```python
from build123d import *

# Parameters (mm, degrees)
SKETCH004_R  = 1.55
PAD005_DEPTH = 0.75
FILLET006_R  = 0.4
FILLET007_R  = 1


with BuildPart() as part:
    # Sketch004 → Pad005 (new body, symmetric)
    with BuildSketch(Plane.XZ):
        with BuildLine():
            Line((-20, 10), (-20, -7))
            Line((-20, -8.5), (-20, -7))
            Line((-20, -8.5), (-20, -10))
            Line((-20, -10), (20, -10))
            Line((20, -10), (20, 4))
            Line((18.133975, 4.5), (20, 4))
            Line((18.133975, 4.5), (-14.2, 4.5))
            ThreePointArc((-15, 4.5), (-14.6, 4.1), (-14.2, 4.5))
            Line((-15, 4.5), (-15, 5.2))
            ThreePointArc((-15, 6), (-15.4, 5.6), (-15, 5.2))
            Line((-15, 6), (18.133975, 6))
            Line((18.133975, 6), (20, 6.5))
            Line((20, 6.5), (20, 10))
            Line((20, 10), (-20, 10))
        make_face()
        Circle(SKETCH004_R, mode=Mode.SUBTRACT)
    extrude(amount=PAD005_DEPTH, both=True)

    # Fillet006
    fillet006_edges = [part.edges().sort_by_distance(p)[0] for p in [
        (-15, 0, 5.2),
        (-14.2, 0, 4.5),
    ]]
    fillet(fillet006_edges, radius=FILLET006_R)

    # Fillet007
    fillet007_edges = [part.edges().sort_by_distance(p)[0] for p in [
        (18.133975, 0, 4.5),
        (18.133975, 0, 6),
        (20, 0, 6.5),
        (20, 0, 10),
        (20, 0, 4),
        (20, 0, -10),
        (-20, 0, -10),
        (-20, 0, 10),
    ]]
    fillet(fillet007_edges, radius=FILLET007_R)


solid = part.part
```
Read the model definition and answer for the solid it produces. Units are mm, in the model's axes. A direction names the side the tool comes from. Coordinates: 2 decimals unless noted, no trailing zeros. Write each loop counter-clockwise with the first axis right and the second up, starting at its lowest first coordinate (ties: lowest second). Pieces come first, ordered by that corner, then holes. Notation, with made-up numbers: (-8.5, 2) -> (40.5, 2) arc R14 cw to (40.5, 15) -> close; hole circle Ø6 at (33.5, -34.75). An arc over 180 degrees is marked (long way). Write item = value, one per line.
(1) Section D-D on x = 16.5 is taken. Write down the section's boundary in (y, z), plus the area to 4 significant figures.
From the geometry:
outline = (-0.75, -10) -> (0.75, -10) -> (0.75, 4.5) -> (-0.75, 4.5) -> close; (-0.75, 6) -> (0.75, 6) -> (0.75, 10) -> (-0.75, 10) -> close
area = 27.75 mm2
(2) Straight lines are drawn through the part: L1, parallel to Z at x = 0, y = 0.1; L2, parallel to Z at x = -7, y = 0.65; L3, parallel to Z at x = -1, y = 0.25. For each, find the intervals that lie inside material, in ascending order. Write a range as from..to.
From the geometry:
L1 = -10..-1.55, 1.55..4.5, 6..10
L2 = -10..4.5, 6..10
L3 = -10..-1.18, 1.18..4.5, 6..10
(3) Which of the six approach directions +Z, -Z, +X, -X, +Y, -Y give full straight-line access (tool end or side, diameter ignored) to faces 5 (the face through (20, 0, 8)), 6 (the face through (19.788, -0.01, 3.849))?
From the geometry:
face_5 = +Z, -Z, +X, +Y, -Y
face_6 = +X, +Y, -Y
(4) Section A-A on z = 0 is taken. Write down the section's boundary in (x, y), plus the area to 4 significant figures.
From the geometry:
outline = (-20, -0.75) -> (-1.55, -0.75) -> (-1.55, 0.75) -> (-20, 0.75) -> close; (1.55, -0.75) -> (20, -0.75) -> (20, 0.75) -> (1.55, 0.75) -> close
area = 55.35 mm2
(5) Given pin 1 Ø2.5 at (x, z) = (0, 0) entering from +Y, flat-ended and moving along its own axis, determine where the tip first touches the part or whether it passes through.
From the geometry:
pin_1 = through
(6) For a pull along Z with two mould halves and no side action, classify faces 1 (the face through (0, 0, -10)), 2 (the face through (2, 0, 4.5)), 3 (the face through (18.753, -0.01, 4.334)), 4 (the face through (0, -0.75, -2)) as +Z half, -Z half, draft (parallel to the pull), parting line (faces both ways), or undercut.
From the geometry:
face_1 = -Z half
face_2 = undercut
face_3 = undercut
face_4 = draft
(7) Section C-C on y = -0.15 is taken. Write down the section's boundary in (x, z).
From the geometry:
outline = (-20, -9) arc R1 ccw to (-19, -10) -> (19, -10) arc R1 ccw to (20, -9) -> (20, 3.23) arc R1 ccw to (19.26, 4.2) -> (18.26, 4.47) arc R1 ccw to (18, 4.5) -> (-13.91, 4.5) arc R0.4 ccw to (-14.25, 4.3) arc R0.4 cw to (-15, 4.5) -> (-15, 4.91) arc R0.4 ccw to (-15.2, 5.25) arc R0.4 cw to (-15, 6) -> (18, 6) arc R1 ccw to (18.26, 6.03) -> (19.26, 6.3) arc R1 ccw to (20, 7.27) -> (20, 9) arc R1 ccw to (19, 10) -> (-19, 10) arc R1 ccw to (-20, 9) -> close; hole circle Ø3.1 at (0, 0)
(8) Section B-B on x = 0 is taken. Write down the section's boundary in (y, z).
From the geometry:
outline = (-0.75, -10) -> (0.75, -10) -> (0.75, -1.55) -> (-0.75, -1.55) -> close; (-0.75, 1.55) -> (0.75, 1.55) -> (0.75, 4.5) -> (-0.75, 4.5) -> close; (-0.75, 6) -> (0.75, 6) -> (0.75, 10) -> (-0.75, 10) -> close
